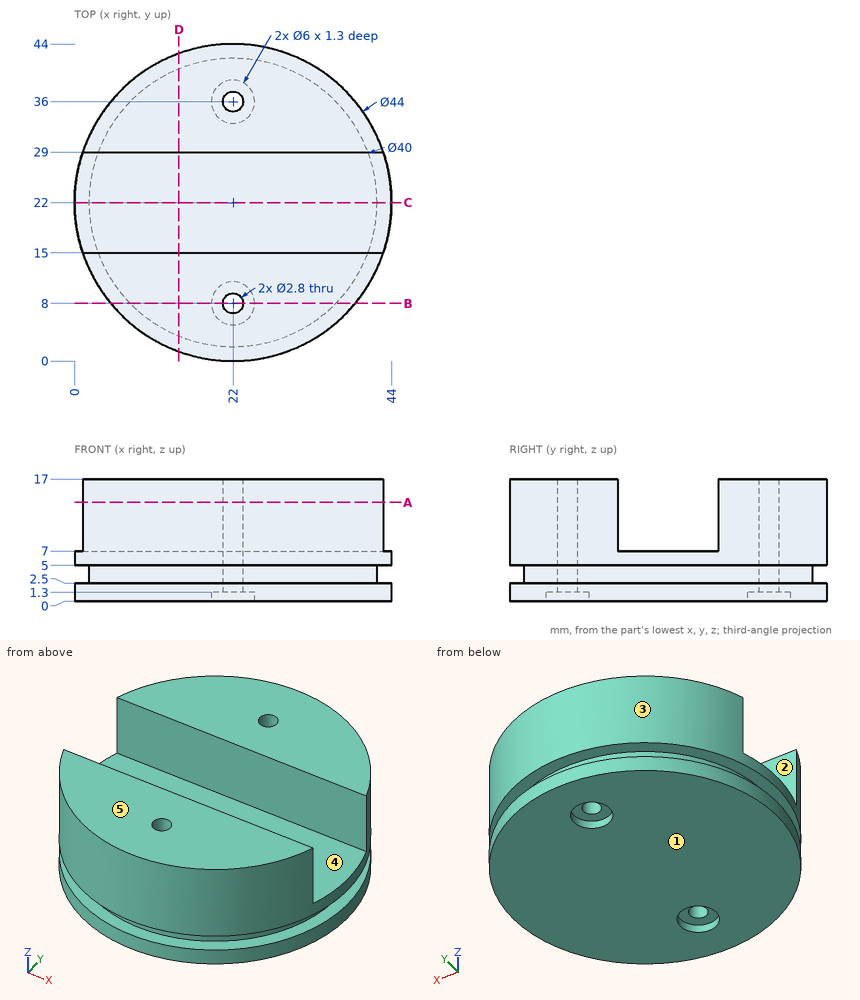
Print and shaded views of the part. All mm, measured from the part's lowest x, y and z. A direction names the side the tool comes from. Give positions to 0.01 mm unless a question says otherwise; leave off trailing zeros. Write each loop counter-clockwise with the first axis right and the second up, starting at its lowest first coordinate (ties: lowest second). Pieces come first, ordered by that corner, then holes. Notation, with made-up numbers: (70, -1.75) -> (79, -1.75) arc R37 ccw to (79, 35.25) -> close; hole circle Ø9 at (24, 10.5). An arc over 180 degrees is marked (long way). Write each question's results on one line, items separated by ' | '.
1. Cut at A-A, the plane z = 13.75. Write the cut outline in (x, y), then the cut area to 3 significant figures.
Geometry check:
outline: (1.14, 15) arc R22 ccw to (42.86, 15) -> close; (1.14, 29) -> (42.86, 29) arc R22 ccw to start; hole circle Ø2.8 at (22, 8); hole circle Ø2.8 at (22, 36) | area: 903 mm²
2. Cut at C-C, the plane y = 22. Write the cut outline in (x, z).
Geometry check:
outline: (0, 0) -> (44, 0) -> (44, 2.5) -> (42, 2.5) -> (42, 5) -> (44, 5) -> (44, 7) -> (0, 7) -> (0, 5) -> (2, 5) -> (2, 2.5) -> (0, 2.5) -> close
3. Cut at B-B, the plane y = 8. Write the cut outline in (x, z), then the cut area to 3 significant figures.
Geometry check:
outline: (5.03, 0) -> (19, 0) -> (19, 1.3) -> (20.6, 1.3) -> (20.6, 17) -> (5.03, 17) -> (5.03, 5) -> (7.72, 5) -> (7.72, 2.5) -> (5.03, 2.5) -> close; (23.4, 1.3) -> (25, 1.3) -> (25, 0) -> (38.97, 0) -> (38.97, 2.5) -> (36.28, 2.5) -> (36.28, 5) -> (38.97, 5) -> (38.97, 17) -> (23.4, 17) -> close | area: 512 mm²
4. Which spindle directions (+Z, -Z, +X, -X, +Y, -Y) get a long thin tool onto all of the face, cutting with end or side? Do the marked faces 4 and 5. Say none if no direction does.
Geometry check:
face 4: +Z, +X, -X | face 5: +Z, +X, -X, +Y, -Y
5. Cut at D-D, the plane x = 14.5. Write the cut outline in (y, z).
Geometry check:
outline: (1.32, 0) -> (42.68, 0) -> (42.68, 2.5) -> (40.54, 2.5) -> (40.54, 5) -> (42.68, 5) -> (42.68, 17) -> (29, 17) -> (29, 7) -> (15, 7) -> (15, 17) -> (1.32, 17) -> (1.32, 5) -> (3.46, 5) -> (3.46, 2.5) -> (1.32, 2.5) -> close
6. Wall check: probe 1 along Y at (x, z) = (22, 0.45); probe 2 along Y at (x, z) = (22, 13); probe 3 along Z at (x, y) = (11, 3.5). Give the ranges that are in metal, low to high. Write a range as [from, to].
Geometry check:
probe 1: [0, 5], [11, 33], [39, 44] | probe 2: [0, 6.6], [9.4, 15], [29, 34.6], [37.4, 44] | probe 3: [0, 2.5], [5, 17]
7. Drop flat-ended pins along their axis: P1, Ø3.5, axis at x = 22, y = 8, coming from the -Z side; P2, Ø1, axis at x = 32, z = 2.5, coming from the +Y side; P3, Ø1.5, axis at x = 34.5, z = 3, coming from the -Y side. Give the stop position or say it passes through.
Geometry check:
P1: z = 1.3 | P2: y = 41.84 | P3: y = 3.52
8. Two-plate mould, pull along Y, no slides. Class the marked faces 1, 2 and 3: pulls with the +Y half, pulls with the -Y half, needs draft (parallel to the pull), parting line crosses it, or undercut.
Geometry check:
face 1: needs draft | face 2: undercut | face 3: parting line crosses it
